```python
from build123d import *

# Parameters (mm, degrees)
EXTRUDE_1_DEPTH     = 40
SKETCH_8_R          = 2
CUT_EXTRUDE_5_DEPTH = 50


with BuildPart() as part:
    # Эскиз1 → Бобышка-Вытянуть1 (new body)
    with BuildSketch(Plane.XY):
        with BuildLine():
            Line((0, 0), (140, 0))
            Line((140, 0), (140, 34))
            Line((140, 34), (140, 50))
            Line((140, 50), (0, 50))
            Line((0, 50), (0, 26))
            Line((0, 26), (12.566965626, 26))
            ThreePointArc((12.566965626, 26), (27.5, 25), (12.566965626, 24))
            Line((12.566965626, 24), (0, 24))
            Line((0, 24), (0, 0))
        make_face()
        with BuildLine():
            Line((62.566965626, 26), (45, 26))
            Line((45, 26), (45, 24))
            Line((45, 24), (62.566965626, 24))
            ThreePointArc((62.566965626, 24), (70, 17.5), (77.433034374, 24))
            Line((77.433034374, 24), (94.997657208, 24))
            Line((94.997657208, 24), (94.997657208, 26))
            Line((94.997657208, 26), (77.433034374, 26))
            ThreePointArc((77.433034374, 26), (70, 32.5), (62.566965626, 26))
        make_face(mode=Mode.SUBTRACT)
    extrude(amount=EXTRUDE_1_DEPTH)

    # Эскиз8 → Вырез-Вытянуть5 (cut)
    with BuildSketch(Plane.XZ):
        with Locations(Location((8, 30, 0), (0, 0, 270))):
            Circle(SKETCH_8_R)
        with Locations(Location((8, 10, 0), (0, 0, 270))):
            Circle(SKETCH_8_R)
        with Locations(Location((55, 30, 0), (0, 0, 270))):
            Circle(SKETCH_8_R)
        with Locations(Location((55, 10, 0), (0, 0, 270))):
            Circle(SKETCH_8_R)
        with Locations(Location((85, 30, 0), (0, 0, 270))):
            Circle(SKETCH_8_R)
        with Locations(Location((85, 10, 0), (0, 0, 270))):
            Circle(SKETCH_8_R)
    extrude(amount=-CUT_EXTRUDE_5_DEPTH, mode=Mode.SUBTRACT)


solid = part.part
```
Here's how the part is built. I have some questions about the finished solid (model axes, mm). A direction names the side the tool comes from. Give positions to 0.01 mm unless a question says otherwise; leave off trailing zeros. Order: outer loops, then holes, each group sorted by start corner. A loop starts at its lowest first (then second) coordinate and runs counter-clockwise, first axis right, second up. Notation, with made-up numbers: (66.25, 0) - (96.25, 0) arc R24 cw to (96.25, 17) - close; hole circle Ø5 at (55, -34). An arc over 180 degrees is marked (long way). Answer as a JSON object with one key per item and string values. Group by question number.
Item 1: If we section it at B-B on z = 34: Please give me the cut outline in (x, y), and give its area (3 significant figures).
Item 2: If we section it at D-D on x = 85: Please give me the cut outline in (y, z).
Item 3: If we section it at A-A on x = 20: Please give me the cut outline in (y, z).
Item 4: Which directions (+Z, -Z, +X, -X, +Y, -Y) give clear straight access to the entire face, cutting with the end or side of a thin tool? Please do faces 1 (the flat face through (6, 24, 20)), 2 (the cylindrical face through (10, 12, 10)), 3 (the flat face through (86, 26, 20)).
Item 5: For P1, Ø2, axis at x = 24.5, y = 28, coming from the +Z side; P2, Ø1, axis at y = 25, z = 24, coming from the -X side, each with a flat end and sliding along its axis, tell me the tip position at first contact or that it passes through.
Item 6: If we section it at C-C on y = 28: Give the number of separate pieces and of enclosed holes in the cut face, and give its area (3 significant figures).
Item 7: If we mould it in two halves opening along Y, with no side actions, what happens to faces 4 (the flat face through (54, 24, 20)), 5 (the cylindrical face through (86.686, 11.832, 28.925))? For each: pulls with the +Y half, pulls with the -Y half, needs draft (parallel to the pull), parting line crosses it, or undercut.
Item 8: Please list where these lines run through material, in increasing order: probe 1 along X at (y, z) = (42, 10); probe 2 along Y at (x, z) = (52, 33.5); probe 3 along Z at (x, y) = (83.5, 9.5).
Result set:
{
 "1": {"outline": "(0, 0) - (140, 0) - (140, 50) - (0, 50) - (0, 26) - (12.57, 26) arc R7.5 cw (long way) to (12.57, 24) - (0, 24) - close; hole (45, 24) - (62.57, 24) arc R7.5 ccw to (77.43, 24) - (95, 24) - (95, 26) - (77.43, 26) arc R7.5 ccw to (62.57, 26) - (45, 26) - close", "area": "6,550 mm²"},
 "2": {"outline": "(0, 0) - (24, 0) - (24, 8) - (0, 8) - close; (0, 12) - (24, 12) - (24, 28) - (0, 28) - close; (0, 32) - (24, 32) - (24, 40) - (0, 40) - close; (26, 0) - (50, 0) - (50, 8) - (26, 8) - close; (26, 12) - (50, 12) - (50, 28) - (26, 28) - close; (26, 32) - (50, 32) - (50, 40) - (26, 40) - close"},
 "3": {"outline": "(0, 0) - (17.5, 0) - (17.5, 40) - (0, 40) - close; (32.5, 0) - (50, 0) - (50, 40) - (32.5, 40) - close"},
 "4": {"face 1": "+Z, -Z, -X", "face 2": "+Y, -Y", "face 3": "+Z, -Z"},
 "5": {"P1": "through", "P2": "x = 27.48"},
 "6": {"separate pieces": "3", "enclosed holes": "6", "area": "4,420 mm²"},
 "7": {"face 4": "undercut", "face 5": "needs draft"},
 "8": {"probe 1": "0 to 6, 10 to 53, 57 to 83, 87 to 140", "probe 2": "0 to 24, 26 to 50", "probe 3": "0 to 8.68, 11.32 to 28.68, 31.32 to 40"}
}
